The figure shows three views and two pictorial views of one solid part (mm, origin at its lowest corner). Answer the questions. Coordinates: 2 decimals unless noted, no trailing zeros. Loops run counter-clockwise (first coordinate to the right, second up) from the corner with the lowest first, then second, coordinate; pieces in that order, holes last. Notation, with made-up numbers: (87, 14) - (120, 14) arc R9 ccw to (120, 26) - close; hole circle Ø5 at (5, 80). An arc over 180 degrees is marked (long way). Return JSON: item names as keys, results as strings. Group by question number.
1. This flat-tipped pin is pushed along its axis until it touches: P1, Ø6, axis at x = 19, z = 13.5, coming from the -Y side. Where does it stop, or does it pass through?
2. Section A-A (z = 36.5) is taken. Write down the section's boundary in (x, y).
3. Find the intervals of material crossed by line 1 along Z through (x, y) = (7.75, 4.8); line 2 along X through (y, z) = (1.7, 8); line 3 along X through (y, z) = (3.65, 5), in increasing order.
4. Section D-D (z = 46.5) is taken. Write down the section's boundary in (x, y), and give its area (3 significant figures).
5. Section C-C (x = 8) is taken. Write down the section's boundary in (y, z), and give its area (3 significant figures).
6. The mould has two halves that part along X. Classify the marked faces 1, 2, 3 and 4: pulls with the +X half, pulls with the -X half, needs draft (parallel to the pull), parting line crosses it, or undercut.
7. Section B-B (y = 0.6) is taken. Write down the section's boundary in (x, z), and give its area (3 significant figures).
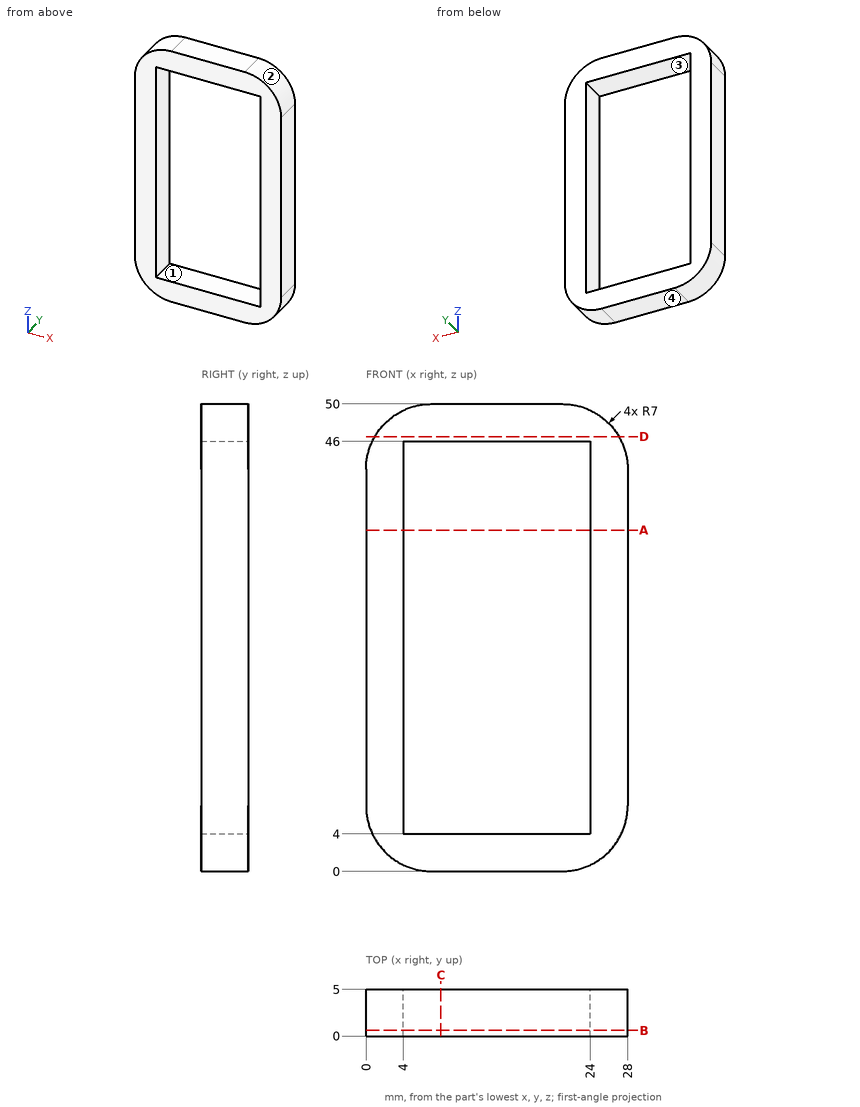
The answers:
{
 "1": {"P1": "passes through"},
 "2": {"outline": "(0, 0) - (4, 0) - (4, 5) - (0, 5) - close; (24, 0) - (28, 0) - (28, 5) - (24, 5) - close"},
 "3": {"line 1": "z = 0 to 4, 46 to 50", "line 2": "x = 0 to 4, 24 to 28", "line 3": "x = 0.29 to 4, 24 to 27.71"},
 "4": {"outline": "(0.94, 0) - (27.06, 0) - (27.06, 5) - (0.94, 5) - close", "area": "131 mm2"},
 "5": {"outline": "(0, 0) - (5, 0) - (5, 4) - (0, 4) - close; (0, 46) - (5, 46) - (5, 50) - (0, 50) - close", "area": "40.0 mm2"},
 "6": {"face 1": "undercut", "face 2": "pulls with the +X half", "face 3": "undercut", "face 4": "needs draft"},
 "7": {"outline": "(0, 7) arc R7 ccw to (7, 0) - (21, 0) arc R7 ccw to (28, 7) - (28, 43) arc R7 ccw to (21, 50) - (7, 50) arc R7 ccw to (0, 43) - close; hole (4, 4) - (24, 4) - (24, 46) - (4, 46) - close", "area": "518 mm2"}
}
